Here's how the part is built. I have some questions about the finished solid (model axes, mm). Face numbers are marked on the shaded views. A direction names the side the tool comes from. Give positions to 0.01 mm unless a question says otherwise; leave off trailing zeros. Order: outer loops, then holes, each group sorted by start corner. A loop starts at its lowest first (then second) coordinate and runs counter-clockwise, first axis right, second up. Notation, with made-up numbers: M 35.25,43.25 L 71.25,43.25 A28 ccw 71.25,64.25 Z; hole C 10.5,-30 d4. An arc over 180 degrees is marked long. Use CSV: the item, a comma, the result in double quotes. Start each with the question number.
```python
from build123d import *

# Parameters (mm, degrees)
SKETCH066_R             = 1.75
PAD046_DEPTH            = 2
SKETCH067_W             = 10
SKETCH067_H             = 2
PAD047_DEPTH            = 10
SKETCH068_W             = 10
SKETCH068_H             = 4
PAD048_DEPTH            = 10
SKETCH069_R             = 1.75
POCKET012_DEPTH         = 4.001
BODY015_PLACEMENT_ANGLE = 180


with BuildPart() as part:
    # Sketch066 → Pad046 (new body)
    with BuildSketch(Plane.XZ):
        with BuildLine():
            Line((-18.7, 6.5), (18.7, 6.5))
            ThreePointArc((18.7, -6.5), (25.2, 0), (18.7, 6.5))
            Line((18.7, -6.5), (-18.7, -6.5))
            ThreePointArc((-18.7, 6.5), (-25.2, 0), (-18.7, -6.5))
        make_face()
        with Locations((-18.7, 0)):
            Circle(SKETCH066_R, mode=Mode.SUBTRACT)
        with Locations((18.7, 0)):
            Circle(SKETCH066_R, mode=Mode.SUBTRACT)
    extrude(amount=PAD046_DEPTH)

    # Sketch067 (on Face1 of Pad046) → Pad047 (join)
    with BuildSketch(Plane(origin=(0, 0, -6.5), x_dir=(1, 0, 0), z_dir=(0, 0, -1))):
        with Locations((0, 1)):
            Rectangle(SKETCH067_W, SKETCH067_H)
    extrude(amount=PAD047_DEPTH)

    # Sketch068 (on Face12 of Pad047) → Pad048 (join)
    with BuildSketch(Plane.XZ.offset(2)):
        with Locations((0, -14.5)):
            Rectangle(SKETCH068_W, SKETCH068_H)
    extrude(amount=PAD048_DEPTH)

    # Sketch069 (on Face16 of Pad048) → Pocket012 (cut, through all)
    with BuildSketch(Plane(origin=(0, 0, -12.5), x_dir=(-1, 0, 0), z_dir=(0, 0, 1))):
        with Locations((0, 7)):
            Circle(SKETCH069_R)
    extrude(amount=-POCKET012_DEPTH, mode=Mode.SUBTRACT)


with BuildPart() as part_1:
    # Body015 placement: moved
    add(part.part.moved(Location((-82.5, 61.5, 20))).rotate(Axis((-82.5, 61.5, 20), (0, 0, 1)), BODY015_PLACEMENT_ANGLE))


solid = part_1.part
```
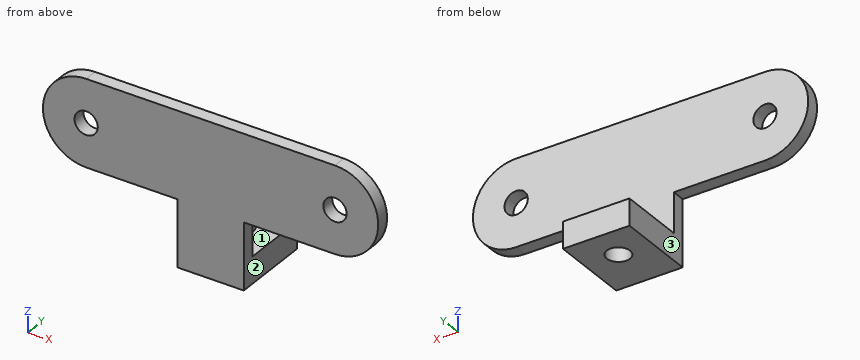
Q1. Imagine slicing it at A-A, the plane x = -82.5. Please give me the cut outline in (y, z).
Q2. Imagine slicing it at B-B, the plane z = 19. Please give me the cut outline in (x, y).
Q3. Imagine slicing it at D-D, the plane x = -70. Please give me the cut outline in (y, z), then the cut area to 3 significant figures.
Q4. For P1, Ø3, axis at x = -101.2, z = 20, coming from the -Y side; P2, Ø3, axis at x = -78.5, y = 68, coming from the +Z side; P3, Ø0.6, axis at x = -69, y = 62, coming from the -Z side, each with a flat end and sliding along its axis, tell me the tip position at first contact or that it passes through.
Q5. For the marked faces 1, 2 and 3, which set-ups out of +Z, -Z, +X, -X, +Y, -Y let a thin tool reach every point of the face, with its end or its side?
Q6. I need wall thicknesses on line 1 (Z direction, x = -63.8, y = 62.55); line 2 (X direction, y = 68.5, z = 6.05); line 3 (X direction, y = 63.25, z = 18.75). Which ranges of each line are inside material? Lowest first, please. Write a range as [from, to].
Q7. Imagine slicing it at C-C, the plane y = 71.75. Please give me the cut outline in (x, z).
Reply:
1,outline,"M 61.5,3.5 L 66.75,3.5 L 66.75,7.5 L 63.5,7.5 L 63.5,26.5 L 61.5,26.5 Z; M 70.25,3.5 L 73.5,3.5 L 73.5,7.5 L 70.25,7.5 Z"
2,outline,"M -107.62,61.5 L -102.64,61.5 L -102.64,63.5 L -107.62,63.5 Z; M -99.76,61.5 L -65.24,61.5 L -65.24,63.5 L -99.76,63.5 Z; M -62.36,61.5 L -57.38,61.5 L -57.38,63.5 L -62.36,63.5 Z"
3,outline,"M 61.5,13.5 L 63.5,13.5 L 63.5,26.5 L 61.5,26.5 Z"
3,area,"26.0 mm^2"
4,P1,"passes through"
4,P2,"stops at z = 7.5"
4,P3,"stops at z = 13.5"
5,face 1,"+Z, +X, -X, +Y"
5,face 2,"-Z, +X, +Y, -Y"
5,face 3,"-Z, -X, +Y, -Y"
6,line 1,"z = [13.5, 18.25], [21.75, 26.5]"
6,line 2,"x = [-87.5, -84.25], [-80.75, -77.5]"
6,line 3,"x = [-107.58, -102.42], [-99.98, -65.02], [-62.58, -57.42]"
7,outline,"M -87.5,3.5 L -77.5,3.5 L -77.5,7.5 L -87.5,7.5 Z"
